Here's how the part is built. I have some questions about the finished solid (model axes, mm). A direction names the side the tool comes from. Round coordinates to 2 decimals unless told otherwise and drop trailing zeros. Write each loop counter-clockwise with the first axis right and the second up, starting at its lowest first coordinate (ties: lowest second). Pieces come first, ordered by that corner, then holes. Notation, with made-up numbers: (16, 46.25) - (58, 46.25) arc R24 cw to (58, 63.25) - close; hole circle Ø9 at (56, -39). An arc over 180 degrees is marked (long way). One line per item, written item: value. Start each with the question number.
Item 1: For P1, Ø1.5, axis at x = 154, z = 1, coming from the +Y side; P2, Ø0.9, axis at x = 281, z = 1, coming from the -Y side, each with a flat end and sliding along its axis, tell me the tip position at first contact or that it passes through.
Item 2: For faces 1 (the face through (6.014, 45.703, 1.521)), 2 (the face through (-44.297, 93.986, 1.521)), 3 (the face through (694.297, -6.014, 1.521)), which set-ups out of +Z, -Z, +X, -X, +Y, -Y let a thin tool reach every point of the face, with its end or its side?
Item 3: Thinking about a two-plate mould opening in X: for faces 4 (the face through (705.703, 93.986, 1.521)), 5 (the face through (-5.703, -53.986, 1.521)), 6 (the face through (-43.986, -54.297, 1.521)), 7 (the face through (743.986, -54.297, 1.521)), which applies, released by +X, released by -X, zero draft, split by the parting line, or undercut?
Item 4: Imagine slicing it at A-A, the plane z = 0.95. Count the separate pieces of the cut face and the enclosed holes in it, then the cut area to 3 significant figures.
Item 5: If I drill on line 1 (Y direction, x = -25, z = 2.2); line 2 (X direction, y = 21, z = 0.45); line 3 (X direction, y = -33, z = 1.15), over which ranges is the centre line in solid material (lowest first)?
Item 6: Imagine slicing it at B-B, the plane x = 630. Please give me the cut outline in (y, z), then the cut area to 3 significant figures.
```python
from build123d import *

# Parameters (mm, degrees)
SKETCH1_W           = 700
SKETCH1_H           = 40
SKETCH1_W_2         = 50
SKETCH1_H_2         = 160
SKETCH1_R           = 5
BOSS_EXTRUDE1_DEPTH = 3
FILLET1_R           = 20
SKETCH2_R           = 4
CUT_EXTRUDE1_DEPTH  = 757.643244865


with BuildPart() as part:
    # Sketch1 → Boss-Extrude1 (new body)
    # profile 1 of 3: a face of its own
    with BuildSketch(Plane.XY):
        with Locations((350, 20)):
            Rectangle(SKETCH1_W, SKETCH1_H)
    # profile 2 of 3: a face of its own
    with BuildSketch(Plane.XY):
        with Locations((-25, 20)):
            Rectangle(SKETCH1_W_2, SKETCH1_H_2)
        with Locations((-25, 80)):
            Circle(SKETCH1_R, mode=Mode.SUBTRACT)
        with Locations((-25, -40)):
            Circle(SKETCH1_R, mode=Mode.SUBTRACT)
    # profile 3 of 3: a face of its own
    with BuildSketch(Plane.XY):
        with Locations((725, 20)):
            Rectangle(SKETCH1_W_2, SKETCH1_H_2)
        with Locations((725, 80)):
            Circle(SKETCH1_R, mode=Mode.SUBTRACT)
        with Locations((725, -40)):
            Circle(SKETCH1_R, mode=Mode.SUBTRACT)
    extrude(amount=BOSS_EXTRUDE1_DEPTH)

    # Fillet1
    fillet1_edges = [part.edges().sort_by_distance(p)[0] for p in [
        (0, 0, 1.5),
        (0, -60, 1.5),
        (-50, -60, 1.5),
        (-50, 100, 1.5),
        (0, 100, 1.5),
        (0, 40, 1.5),
        (700, 40, 1.5),
        (700, 100, 1.5),
        (750, 100, 1.5),
        (750, -60, 1.5),
        (700, -60, 1.5),
        (700, 0, 1.5),
    ]]
    fillet(fillet1_edges, radius=FILLET1_R)

    # Sketch2 → Cut-Extrude1 (cut, through all)
    with BuildSketch(Plane.XY.offset(3)):
        with Locations((-25, 45)):
            Circle(SKETCH2_R)
        with Locations((-25, -5)):
            Circle(SKETCH2_R)
        with Locations((-25, 20)):
            Circle(SKETCH2_R)
        with Locations(Location((725, 20, 0), (0, 0, 180))):
            Circle(SKETCH2_R)
        with Locations(Location((725, -5, 0), (0, 0, 180))):
            Circle(SKETCH2_R)
        with Locations(Location((725, 45, 0), (0, 0, 180))):
            Circle(SKETCH2_R)
    extrude(amount=-CUT_EXTRUDE1_DEPTH, mode=Mode.SUBTRACT)


solid = part.part
```
Values follow:
1. P1: stops at y = 40
1. P2: stops at y = 0
2. face 1: +Z, -Z, +Y
2. face 2: +Z, -Z, -X, +Y
2. face 3: +Z, -Z, -Y
3. face 4: undercut
3. face 5: undercut
3. face 6: released by -X
3. face 7: released by +X
4. separate pieces: 1
4. enclosed holes: 10
4. area: 43,000 mm^2
5. line 1: y = -60 to -45, -35 to -9, -1 to 16, 24 to 41, 49 to 75, 85 to 100
5. line 2: x = -50 to -28.87, -21.13 to 721.13, 728.87 to 750
5. line 3: x = -50 to 0, 700 to 750
6. outline: (0, 0) - (40, 0) - (40, 3) - (0, 3) - close
6. area: 120 mm^2
